from build123d import *

# Parameters (mm, degrees)
CROQUIS1_R              = 8.25
CROQUIS1_R_2            = 4.25
SALIENTE_EXTRUIR1_DEPTH = 2
CROQUIS2_R              = 5.5
CROQUIS2_R_2            = 4.25
SALIENTE_EXTRUIR2_DEPTH = 4.5


with BuildPart() as part:
    # Croquis1 → Saliente-Extruir1 (new body)
    with BuildSketch(Plane.XY):
        Circle(CROQUIS1_R)
        Circle(CROQUIS1_R_2, mode=Mode.SUBTRACT)
    extrude(amount=-SALIENTE_EXTRUIR1_DEPTH)

    # Croquis2 → Saliente-Extruir2 (add)
    with BuildSketch(Plane(origin=(0, 0, -2), x_dir=(-1, 0, 0), z_dir=(0, 0, -1))):
        with Locations(Location((0, 0, 0), (0, 0, 180))):
            Circle(CROQUIS2_R)
        with Locations(Location((0, 0, 0), (0, 0, 180))):
            Circle(CROQUIS2_R_2, mode=Mode.SUBTRACT)
    extrude(amount=SALIENTE_EXTRUIR2_DEPTH)


solid = part.part
CAD build for the part. Positions are in the model's coordinates, mm. A direction names the side the tool comes from. Give positions to 0.01 mm unless a question says otherwise; leave off trailing zeros. Write each loop counter-clockwise with the first axis right and the second up, starting at its lowest first coordinate (ties: lowest second). Pieces come first, ordered by that corner, then holes. Notation, with made-up numbers: (22.5, 3) -> (78.5, 3) arc R18 cw to (78.5, 24) -> close; hole circle Ø3 at (43.25, 8.25). An arc over 180 degrees is marked (long way). Return JSON: item names as keys, results as strings.
Item 1: Tool access for faces 1 (the flat face through (5.4, -1.7, -2)), 2 (the cylindrical face through (7.62, -3.16, -0.99)): list every direction of +Z, -Z, +X, -X, +Y, -Y with a clear straight run to the whole face (end or side of a thin tool).
Answer below:
{"face 1": "-Z", "face 2": "+Z, -Z"}
Item 2: Band-saw the part on C-C (z = -1.25). List the corners of the cut face in (x, y), then the cut area to 3 significant figures.
Answer below:
{"outline": "circle Ø16.5 at (0, 0); hole circle Ø8.5 at (0, 0)", "area": "157 mm2"}
Item 3: Drill centre lines: probe 1 along Y at (x, z) = (0, -3.8); probe 2 along Y at (x, z) = (0, -1.4); probe 3 along X at (y, z) = (-3.75, -2.5). Where is each one in solid material? Low to high.
Answer below:
{"probe 1": "y = -5.5 to -4.25, 4.25 to 5.5", "probe 2": "y = -8.25 to -4.25, 4.25 to 8.25", "probe 3": "x = -4.02 to -2, 2 to 4.02"}
Item 4: Band-saw the part on A-A (y = 0). List the corners of the cut face in (x, z).
Answer below:
{"outline": "(-8.25, -2) -> (-5.5, -2) -> (-5.5, -6.5) -> (-4.25, -6.5) -> (-4.25, 0) -> (-8.25, 0) -> close; (4.25, -6.5) -> (5.5, -6.5) -> (5.5, -2) -> (8.25, -2) -> (8.25, 0) -> (4.25, 0) -> close"}
Item 5: Drop flat-ended pins along their axis: pin 1 (6 mm diameter, centred on x = 0, y = -3.5, fed in from -Z); pin 2 (1 mm diameter, centred on y = -6, z = -1.5, fed in from -X); pin 3 (7 mm diameter, centred on x = 0, y = 0, fed in from -Z); pin 4 (3 mm diameter, centred on y = 2, z = -1.5, fed in from -X). Give the stop position or say it passes through.
Answer below:
{"pin 1": "stops at z = -6.5", "pin 2": "stops at x = -6.15", "pin 3": "passes through", "pin 4": "stops at x = -8.23"}
Item 6: Band-saw the part on D-D (y = -4.5). List the corners of the cut face in (x, z), then the cut area to 3 significant figures.
Answer below:
{"outline": "(-6.91, -2) -> (-3.16, -2) -> (-3.16, -6.5) -> (3.16, -6.5) -> (3.16, -2) -> (6.91, -2) -> (6.91, 0) -> (-6.91, 0) -> close", "area": "56.1 mm2"}
